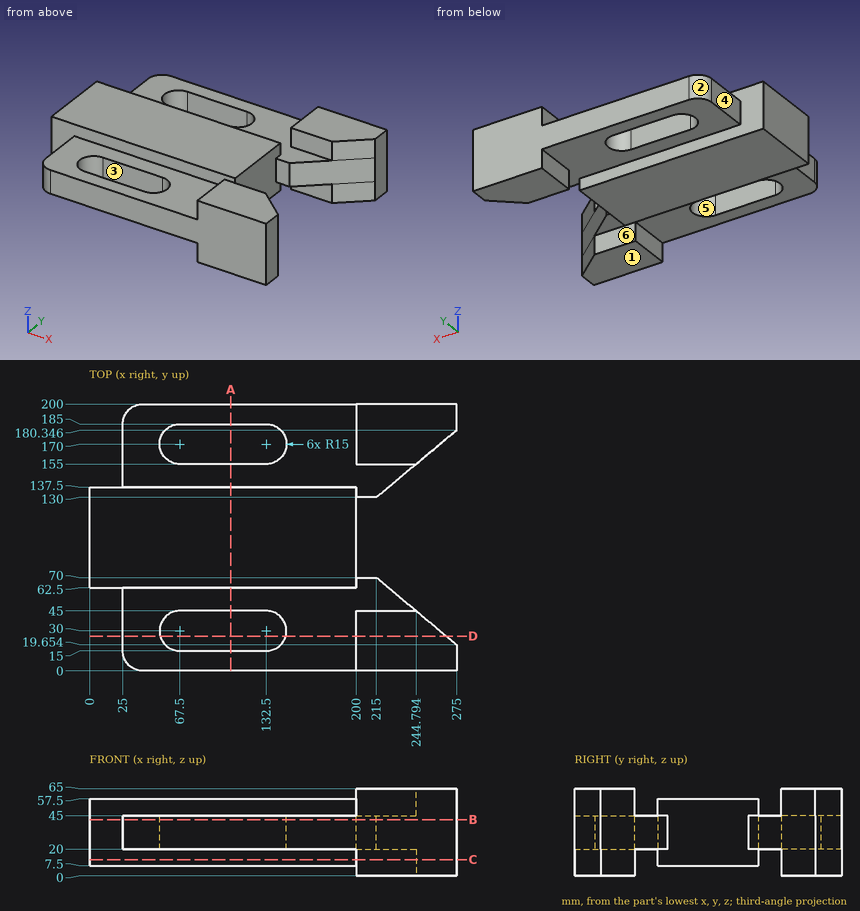
The figure shows three views and two pictorial views of one solid part (mm, origin at its lowest corner). Answer the questions. A direction names the side the tool comes from. Round coordinates to 2 decimals unless told otherwise and drop trailing zeros. Write each loop counter-clockwise with the first axis right and the second up, starting at its lowest first coordinate (ties: lowest second). Pieces come first, ordered by that corner, then holes. Notation, with made-up numbers: (-33.75, -39.75) - (15.25, -39.75) arc R30 ccw to (15.25, -2.75) - close; hole circle Ø4 at (3, -40). An arc over 180 degrees is marked (long way). One line per question, with ' | ' between items. Start each with the question number.
1. Section A-A (x = 106) is taken. Determine the outline of the cut face in (y, z).
2. For a pull along Y with two mould halves and no side action, classify the marked faces 1, 2 and 3 as +Y half, -Y half, draft (parallel to the pull), parting line (faces both ways), or undercut.
3. For the marked faces 4, 5 and 6, determine the directions among +Z, -Z, +X, -X, +Y, -Y from which every point of the face is accessible in a straight line to the end or side of a thin tool.
4. Section B-B (z = 42) is taken. Determine the outline of the cut face in (x, y), and give its area (3 significant figures).
5. Section C-C (z = 12) is taken. Determine the outline of the cut face in (x, y).
6. Section D-D (y = 26) is taken. Determine the outline of the cut face in (x, z), and give its area (3 significant figures).
7. Find the intervals of material crossed by probe 1 along Y at (x, z) = (104, 30); probe 2 along Y at (x, z) = (237, 8.5); probe 3 along Z at (x, y) = (49, 86), in increasing order. Write a range as [from, to].
8. Each of these flat-tipped pins is pushed along its axis until it touches: pin 1 (1.5 mm diameter, centred on y = 134, z = 29.5, fed in from +X); pin 2 (25 mm diameter, centred on y = 85, z = 26.5, fed in from +X); pin 3 (12.5 mm diameter, centred on y = 169, z = 26.5, fed in from -X). Where does it stop, or does it pass through?
Filled in:
1) outline: (0, 20) - (15, 20) - (15, 45) - (0, 45) - close; (45, 20) - (62.5, 20) - (62.5, 7.5) - (137.5, 7.5) - (137.5, 20) - (155, 20) - (155, 45) - (137.5, 45) - (137.5, 57.5) - (62.5, 57.5) - (62.5, 45) - (45, 45) - close; (185, 20) - (200, 20) - (200, 45) - (185, 45) - close
2) face 1: draft | face 2: +Y half | face 3: undercut
3) face 4: +Z, -Z, -X, +Y | face 5: +Z, -Z | face 6: -Z, +X, -X
4) outline: (0, 62.5) - (25, 62.5) - (25, 15) arc R15 ccw to (40, 0) - (275, 0) - (275, 19.65) - (215, 70) - (200, 70) - (200, 130) - (215, 130) - (275, 180.35) - (275, 200) - (40, 200) arc R15 ccw to (25, 185) - (25, 137.5) - (0, 137.5) - close; hole (67.5, 15) - (132.5, 15) arc R15 ccw to (132.5, 45) - (67.5, 45) arc R15 ccw to start; hole (67.5, 155) - (132.5, 155) arc R15 ccw to (132.5, 185) - (67.5, 185) arc R15 ccw to start | area: 38,900 mm²
5) outline: (0, 62.5) - (200, 62.5) - (200, 137.5) - (0, 137.5) - close; (200, 0) - (275, 0) - (275, 19.65) - (244.79, 45) - (200, 45) - close; (200, 155) - (244.79, 155) - (275, 180.35) - (275, 200) - (200, 200) - close
6) outline: (25, 20) - (53.04, 20) - (53.04, 45) - (25, 45) - close; (146.96, 20) - (200, 20) - (200, 0) - (267.44, 0) - (267.44, 65) - (200, 65) - (200, 45) - (146.96, 45) - close | area: 6,410 mm²
7) probe 1: [0, 15], [45, 155], [185, 200] | probe 2: [0, 45], [155, 200] | probe 3: [7.5, 57.5]
8) pin 1: x = 220.66 | pin 2: x = 200 | pin 3: x = 25
